The listing builds one solid part. Answer for the finished solid, in the listing's coordinates (mm). Round coordinates to 2 decimals unless told otherwise and drop trailing zeros. Write each loop counter-clockwise with the first axis right and the second up, starting at its lowest first coordinate (ties: lowest second). Pieces come first, ordered by that corner, then holes. Notation, with made-up numbers: (26, 40.25) - (37, 40.25) arc R25 cw to (37, 63.25) - close; hole circle Ø11 at (-35.5, 52.5). An arc over 180 degrees is marked (long way). Return JSON: item names as keys, results as strings. Group by question number.
(1) Section D-D, the plane z = 1.5 is taken. Give the number of separate pieces and of enclosed holes in the cut face, then the cut area to 3 significant figures.
(2) Section A-A, the plane y = 45 is taken. Write down the section's boundary in (x, z), then the cut area to 3 significant figures.
(3) Section B-B, the plane x = 47 is taken. Write down the section's boundary in (y, z).
(4) Section C-C, the plane y = 105 is taken. Write down the section's boundary in (x, z).
(5) Each of these flat-tipped pins is pushed along its axis until it touches: pin 1 (5 mm diameter, centred on x = 85, y = 17, fed in from -Z); pin 2 (0.9 mm diameter, centred on x = 92, z = 1, fed in from -Y). Where does it stop, or does it pass through?
(6) Find the intervals of material crossed by line 1 along Y through (x, z) = (70, 1.9); line 2 along Y through (x, z) = (82.5, 0.8); line 3 along Y through (x, z) = (87.5, 0.85), in increasing order. Write a range as [from, to].
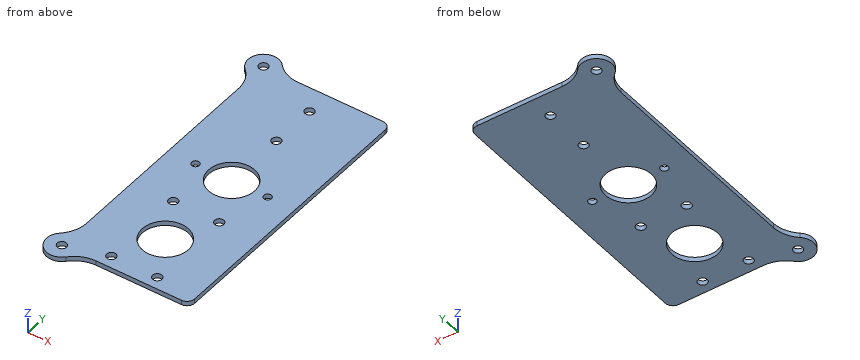
Autodesk Fusion 360 part; units mm, degrees
sketch "Sketch1" plane through (0, 0, 0) normal (0, 0, 1) x (1, 0, 0)
  line L0 (99.5, 80) -> (40.5, 80)
  line L1 (40.5, 80) -> (40.5, 10)
  line L2 (40.5, 10) -> (99.5, 10)
  line L3 (99.5, 10) -> (99.5, 80)
  line L4 (99.5, 80) -> (40.5, 10) construction
  line L5 (40.5, 80) -> (99.5, 10) construction
  line L6 (40.5, 73) -> (100, 73) construction
  line L7 (70, 45) -> (70, 80) construction
  circle A0 centre (55, 73) radius 3
  circle A1 centre (85, 73) radius 3
  line L8 (70, 45) -> (40, 45) construction
  circle A2 centre (55, 17) radius 3
  circle A3 centre (85, 17) radius 3
  circle A4 centre (70, 45) radius 15
  line L9 (101.5, 127.5) -> (38.5, 82.5) construction
  line L10 (101.5, 82.5) -> (38.5, 127.5) construction
  line L11 (101.5, 127.5) -> (38.5, 127.5)
  line L12 (101.5, 82.5) -> (101.5, 127.5)
  line L13 (38.5, 82.5) -> (101.5, 82.5)
  line L14 (38.5, 127.5) -> (38.5, 82.5)
  circle A5 centre (46.5, 105) radius 2.5
  circle A6 centre (70, 105) radius 15
  circle A7 centre (93.5, 105) radius 2.5
  line L15 (70, 80) -> (70, 120) construction
  line L16 (45.0759, 190.4025) -> (95.0759, 190.4025)
  line L17 (95.0759, 190.4025) -> (95.0759, 130.4025)
  line L18 (95.0759, 130.4025) -> (45.0759, 130.4025)
  line L19 (45.0759, 130.4025) -> (45.0759, 190.4025)
  line L20 (70.0759, 190.4025) -> (70.0759, 130.4025) construction
  line L21 (70.0759, 160.4025) -> (95.0759, 160.4025) construction
  circle A8 centre (70.0759, 175.4025) radius 3
  circle A9 centre (70.0759, 145.4025) radius 3
  line L22 (28.5, 191.4025) -> (28.5, 9)
  line L23 (111.5, 191.4025) -> (111.5, 9)
  line L24 (28.5, 191.4025) -> (111.5, 191.4025)
  line L25 (28.5, 9) -> (111.5, 9)
  circle A10 centre (28.5, 191.4025) radius 3
  circle A11 centre (28.5, 191.4025) radius 10
  circle A12 centre (28.5, 9) radius 3
  circle A13 centre (28.5, 9) radius 10
  point P0 (70, 45)
  dimension "d1" = 59
  dimension "d2" = 70
  dimension "d3" = 7
  dimension "d5" = 6
  dimension "d6" = 15
  dimension "d7" = 30
  dimension "d8" = 45
  dimension "d9" = 63
  dimension "d10" = 5
  dimension "d11" = 30
  dimension "d12" = 50
  dimension "d13" = 60
  dimension "d14" = 6
  dimension "d15" = 15
  dimension "d16" = 10
  dimension "d17" = 10
  dimension "d18" = 1
  dimension "d19" = 1
  dimension "d22" = 6
  dimension "d23" = 20
  dimension "d24" = 6
  dimension "d25" = 20
extrude "Extrude1" add sketch "Sketch1" along normal blind 3 contours L0 L1 L2 L3 | L11 L12 L13 L14 | L16 L17 L18 L19 | L22 L24 A10 A11 | L22 L24 A10 A11 | L22 L23 L24 L25 A11 A13 | L22 L25 A12 A13 | L22 L25 A12 A13
fillet "Fillet1" radius 20 2 edges at (38.5, 191.4025, 1.5) (28.5, 181.4025, 1.5)
fillet "Fillet2" radius 20 2 edges at (38.5, 9, 1.5) (28.5, 19, 1.5)
fillet "Fillet3" radius 5 2 edges at (111.5, 191.4025, 1.5) (111.5, 9, 1.5)
equation "d17 = d16"
Working result:
{
 "1": {"separate pieces": "1", "enclosed holes": "12", "area": "14,000 mm^2"},
 "2": {"outline": "(28.5, 0) - (55, 0) - (55, 3) - (28.5, 3) - close; (85, 0) - (111.5, 0) - (111.5, 3) - (85, 3) - close", "area": "159 mm^2"},
 "3": {"outline": "(8.62, 0) - (102.55, 0) - (102.55, 3) - (8.62, 3) - close; (107.45, 0) - (191.78, 0) - (191.78, 3) - (107.45, 3) - close"},
 "4": {"outline": "(28.5, 0) - (44, 0) - (44, 3) - (28.5, 3) - close; (49, 0) - (55, 0) - (55, 3) - (49, 3) - close; (85, 0) - (91, 0) - (91, 3) - (85, 3) - close; (96, 0) - (111.5, 0) - (111.5, 3) - (96, 3) - close"},
 "5": {"pin 1": "passes through", "pin 2": "stops at y = 9"},
 "6": {"line 1": "y = [9, 30], [60, 90], [120, 142.4], [148.4, 172.4], [178.4, 191.4]", "line 2": "y = [9, 15.34], [18.66, 36.71], [53.29, 71.34], [74.66, 96.71], [113.29, 191.4]", "line 3": "y = [9, 15.34], [18.66, 71.34], [74.66, 191.4]"}
}
